```python
from build123d import *

# Parameters (mm, degrees)
ESTRUSIONE_ESTRUSIONE1_DEPTH = 20
SCHIZZO2_W                   = 12
SCHIZZO2_H                   = 25
TAGLIO_ESTRUSIONE1_DEPTH     = 7
SCHIZZO3_R                   = 8
ESTRUSIONE_ESTRUSIONE2_DEPTH = 8
ESTRUSIONE_ESTRUSIONE3_DEPTH = 46
ESTRUSIONE_ESTRUSIONE5_DEPTH = 14
SCHIZZO6_R                   = 6.5
ESTRUSIONE_ESTRUSIONE6_DEPTH = 8
SCHIZZO7_R                   = 3
TAGLIO_ESTRUSIONE2_DEPTH     = 40


with BuildPart() as part:
    # Schizzo1 → Estrusione-Estrusione1 (new body, symmetric)
    with BuildSketch(Plane.XY):
        Polygon((0, 33), (6, 33), (6, -33), (-6, -33), (-6, -3), align=None)
    extrude(amount=ESTRUSIONE_ESTRUSIONE1_DEPTH, both=True)

    # Schizzo2 → Taglio-Estrusione1 (cut)
    with BuildSketch(Plane.XY.offset(20)):
        with Locations((0, -20.5)):
            Rectangle(SCHIZZO2_W, SCHIZZO2_H)
    taglio_estrusione1 = extrude(amount=-TAGLIO_ESTRUSIONE1_DEPTH, mode=Mode.SUBTRACT)

    # Specchia1: Taglio-Estrusione1 across plane
    add(taglio_estrusione1.mirror(Plane.XY), mode=Mode.SUBTRACT)

    # Schizzo3 → Estrusione-Estrusione2 (add)
    with BuildSketch(Plane(origin=(6, 0, 0), x_dir=(0, 0, -1), z_dir=(1, 0, 0))):
        with Locations((0, 6)):
            Circle(SCHIZZO3_R)
    extrude(amount=ESTRUSIONE_ESTRUSIONE2_DEPTH)

    # Schizzo4 → Estrusione-Estrusione3 (add)
    with BuildSketch(Plane(origin=(14, 0, 0), x_dir=(0, 0, -1), z_dir=(1, 0, 0))):
        with BuildLine():
            Line((-14, 6), (-14, -8))
            Line((-14, -8), (14, -8))
            Line((14, -8), (14, 6))
            ThreePointArc((14, 6), (0, 20), (-14, 6))
        make_face()
    extrude(amount=ESTRUSIONE_ESTRUSIONE3_DEPTH)

    # Schizzo5 → Estrusione-Estrusione5 (add)
    with BuildSketch(Plane(origin=(0, 6, 0), x_dir=(1, 0, 0), z_dir=(0, 1, 0))):
        with BuildLine():
            Line((14, -14), (60, -14))
            Line((60, -14), (43.874010565, -29.262780374))
            ThreePointArc((43.874010565, -29.262780374), (37, -32), (30.125989435, -29.262780374))
            Line((30.125989435, -29.262780374), (14, -14))
        make_face()
    estrusione_estrusione5 = extrude(amount=-ESTRUSIONE_ESTRUSIONE5_DEPTH)

    # Specchia2: Estrusione-Estrusione5 across plane
    add(estrusione_estrusione5.mirror(Plane.XY))

    # Schizzo6 → Estrusione-Estrusione6 (add)
    with BuildSketch(Plane(origin=(60, 0, 0), x_dir=(0, 0, -1), z_dir=(1, 0, 0))):
        with Locations((0, 6)):
            Circle(SCHIZZO6_R)
    extrude(amount=ESTRUSIONE_ESTRUSIONE6_DEPTH)

    # Schizzo7 → Taglio-Estrusione2 (cut, through all)
    with BuildSketch(Plane(origin=(0, 6, 0), x_dir=(1, 0, 0), z_dir=(0, 1, 0))):
        with Locations((37, -22)):
            Circle(SCHIZZO7_R)
    taglio_estrusione2 = extrude(amount=-TAGLIO_ESTRUSIONE2_DEPTH, mode=Mode.SUBTRACT)

    # Specchia3: Taglio-Estrusione2 across plane
    add(taglio_estrusione2.mirror(Plane.XY), mode=Mode.SUBTRACT)


solid = part.part
```
Design review of the part built by this model. Coordinates are the model's own, in mm. A direction names the side the tool comes from. Coordinates: 2 decimals unless noted, no trailing zeros. Order: outer loops, then holes, each group sorted by start corner. A loop starts at its lowest first (then second) coordinate and runs counter-clockwise, first axis right, second up. Notation, with made-up numbers: (83.25, 59.25) -> (137.25, 59.25) arc R29 ccw to (137.25, 92.25) -> close; hole circle Ø4 at (-10.75, -17.5). An arc over 180 degrees is marked (long way). One line per item, written item: value. Start each with the question number.
Q1. Insertion check: pin 1 Ø7 at (x, z) = (37, 22) entering from -Y; pin 2 Ø5.5 at (x, z) = (37, -22) entering from -Y; pin 3 Ø9 at (x, z) = (42, -22.5) entering from +Y; pin 4 Ø6 at (x, y) = (1, 18) entering from -Z. Each pin has a flat end and moves straight along its axis. Give the tip position at first contact, or say it passes through.
Q2. Take a section at C-C, the plane x = 37.5. State the section outline as (y, z) points, then the cut area to 3 significant figures.
Q3. Take a section at D-D, the plane z = 0. State the section outline as (x, y) points, then the cut area to 3 significant figures.
Q4. For probe 1 along Z at (x, y) = (37, 0); probe 2 along X at (y, z) = (-2, 22); probe 3 along Z at (x, y) = (1, 15.5), list the stretches that pass through material, from the lowest coordinate up.
Q5. Take a section at B-B, the plane y = 16.5. State the section outline as (x, z) points.
Q6. Mouldability with a two-part tool opening along X and no side actions: class faces 6 (the flat face through (68, 6, 0)), 7 (the flat face through (0, -8, -17)), 8 (the flat face through (14, 0, -6)) as pulls with the +X half, pulls with the -X half, needs draft (parallel to the pull), parting line crosses it, or undercut.
Q7. Take a section at A-A, the plane z = 23.5. State the section outline as (x, y) points.
Q8. Tool access review of faces 1 (the cylindrical face through (63.944, 2.045, 5.158)), 2 (the flat face through (1, 8, 20)), 3 (the flat face through (22.18, -0.9, -21.74)), 4 (the cylindrical face through (9.94, -1.81, 1.73)), 5 (the flat face through (0, -20, 13)): name each direction out of +Z, -Z, +X, -X, +Y, -Y from which nothing blocks a thin tool from reaching the whole face with its end or side.
Values follow:
1. pin 1: stops at y = -8
1. pin 2: passes through
1. pin 3: stops at y = 6
1. pin 4: stops at z = -20
2. outline: (-8, -31.99) -> (6, -31.99) -> (6, -24.96) -> (-8, -24.96) -> close; (-8, -19.04) -> (6, -19.04) -> (6, -14) arc R14 ccw to (6, 14) -> (6, 19.04) -> (-8, 19.04) -> close; (-8, 24.96) -> (6, 24.96) -> (6, 31.99) -> (-8, 31.99) -> close
2. area: 1,040 mm2
3. outline: (-6, -33) -> (6, -33) -> (6, -2) -> (14, -2) -> (14, -8) -> (60, -8) -> (60, -0.5) -> (68, -0.5) -> (68, 12.5) -> (60, 12.5) -> (60, 20) -> (14, 20) -> (14, 14) -> (6, 14) -> (6, 33) -> (0, 33) -> (-6, -3) -> close
3. area: 2,200 mm2
4. probe 1: z = -32 to -25, -19 to 19, 25 to 32
4. probe 2: x = 22.45 to 34, 40 to 51.55
4. probe 3: z = -20 to 20
5. outline: (-2.75, -20) -> (6, -20) -> (6, 20) -> (-2.75, 20) -> close; (14, -9.26) -> (60, -9.26) -> (60, 9.26) -> (14, 9.26) -> close
6. face 6: pulls with the +X half
6. face 7: needs draft
6. face 8: undercut
7. outline: (24.04, -8) -> (34.4, -8) -> (34.4, 6) -> (24.04, 6) -> close; (39.6, -8) -> (49.96, -8) -> (49.96, 6) -> (39.6, 6) -> close
8. face 1: +X
8. face 2: +Z, -X, +Y, -Y
8. face 3: -Z, +Y, -Y
8. face 4: none
8. face 5: +Z, +X, -X, -Y
